Autodesk Inventor part; units mm, degrees
ref_plane "YZ Plane" through (0, 0, 0) normal (1, 0, 0) x (0, 1, 0)
ref_plane "XZ Plane" through (0, 0, 0) normal (0, 1, 0) x (-1, 0, 0)
ref_plane "XY Plane" through (0, 0, 0) normal (0, 0, 1) x (1, 0, 0)
sketch "Boceto2" plane through (0, 0, 0) normal (1, 0, 0) x (0, 1, 0)
  line L0 (-0.2, 0) -> (-0.2, -0.62)
  line L1 (-0.2, -0.62) -> (-0.99, -1.0761)
  line L2 (-0.99, -1.0761) -> (-0.99, -11.1361)
  line L3 (-0.99, -11.1361) -> (0, -11.1361)
  line L4 (0, 0) -> (-0.2, 0)
  line L5 (0, -11.1361) -> (0, 0)
  dimension "d10" = 0.2
  dimension "d11" = 0.62
  dimension "d12" = 10.06
  dimension "d13" = 60
  dimension "d14" = 0.99
extrude "Extrusión1" add sketch "Boceto2" along normal blind 0.1
mirror "Simetría1" about plane through (0, 0, -11.1361) normal (0, 1, 0) of "Extrusión1"
equation "\"d10\" = 0.5 * d18"
equation "\"d11\" = d15"
equation "\"d12\" = d16"
equation "\"d13\" = d17"
equation "\"d14\" = 0.5 * d19"
equation "\"Dc\" = 0.4"
equation "\"Lc\" = 0.62"
equation "\"Ln\" = 10.06"
equation "\"Do\" = 1.98"
equation "\"alfa\" = 60deg"
equation "\"d15\" = 0.62"
equation "\"d16\" = 10.06"
equation "\"d17\" = 60deg"
equation "\"d18\" = 0.4"
equation "\"d19\" = 1.98"
properties part number "2DBoquilla0.4"
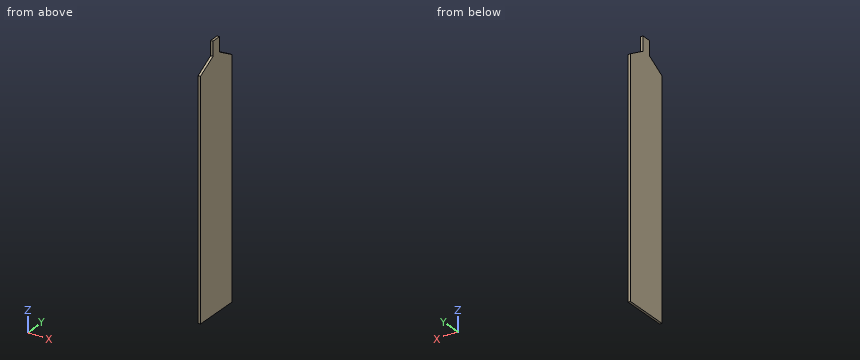
Read the model definition and answer for the solid it produces. Units are mm, in the model's axes. Give positions to 0.01 mm unless a question says otherwise; leave off trailing zeros. Write each loop counter-clockwise with the first axis right and the second up, starting at its lowest first coordinate (ties: lowest second). Pieces come first, ordered by that corner, then holes. Notation, with made-up numbers: (-38.75, -22.75) - (-33.75, -22.75) arc R14 cw to (-33.75, -17.75) - close; hole circle Ø7 at (62.25, -40). An arc over 180 degrees is marked (long way). Use CSV: the item, a comma, the result in double quotes. Start each with the question number.
(1) Consider line 1 along Z through (x, y) = (0.05, 0.8). Determine where the line is inside the solid, lowest interval first.
(2) Find section A-A (x = 0.05). Give the vertices of the cut face in (y, z).
(3) Find section B-B (y = -0.5). Give the vertices of the cut face in (x, z), plus the area to 3 significant figures.
(4) Find section C-C (y = 0.4). Give the vertices of the cut face in (x, z), plus the area to 3 significant figures.
Findings below:
1,line 1,"-11.14 to -0.97"
2,outline,"(-0.99, -11.14) - (0.99, -11.14) - (0.99, -1.08) - (0.2, -0.62) - (0.2, 0) - (-0.2, 0) - (-0.2, -0.62) - (-0.99, -1.08) - close"
3,outline,"(0, -11.14) - (0.1, -11.14) - (0.1, -0.79) - (0, -0.79) - close"
3,area,"1.03 mm2"
4,outline,"(0, -11.14) - (0.1, -11.14) - (0.1, -0.74) - (0, -0.74) - close"
4,area,"1.04 mm2"
